from build123d import *

# Parameters (mm, degrees)
SKETCH2_R          = 4.445
CUT_EXTRUDE1_DEPTH = 18.034
CHAMFER1_SIZE      = 0.762
SKETCH5_W          = 11.240575932
SKETCH5_H          = 1.524
CUT_EXTRUDE2_DEPTH = 20.444017921
CIRPATTERN1_COUNT  = 4


with BuildPart() as part:
    # Sketch1 → Revolve1 (revolve)
    with BuildSketch(Plane.XY, mode=Mode.PRIVATE) as revolve1_sk:
        with BuildLine():
            Line((0, 0), (15.939575932, 0))
            Line((15.939575932, 0), (15.939575932, 6.251377289))
            ThreePointArc((15.939575932, 6.251377289), (15.12834599, 7.110581459), (14.224, 6.35))
            Line((14.224, 6.35), (1.524, 6.35))
            Line((1.524, 6.35), (1.524, 7.874))
            Line((1.524, 7.874), (0, 7.874))
            Line((0, 7.874), (0, 0))
        make_face()
    revolve(revolve1_sk.sketch.rotate(Axis((0, 0, 0), (1, 0, 0)), 90), axis=Axis((0, 0, 0), (1, 0, 0)))

    # Sketch2 → Cut-Extrude1 (cut)
    with BuildSketch(Plane.ZY):
        Circle(SKETCH2_R)
    extrude(amount=-CUT_EXTRUDE1_DEPTH, mode=Mode.SUBTRACT)

    # Chamfer1
    chamfer1_edges = [part.edges().sort_by_distance(p)[0] for p in [
        (15.939575932, 0, -4.445),
        (0, 0, -4.445),
    ]]
    chamfer(chamfer1_edges, length=CHAMFER1_SIZE)

    # Sketch5 → Cut-Extrude2 (cut, through all)
    with BuildSketch(Plane.XY):
        with Locations((10.319287966, 0)):
            Rectangle(SKETCH5_W, SKETCH5_H)
    cut_extrude2 = extrude(amount=-CUT_EXTRUDE2_DEPTH, mode=Mode.SUBTRACT)

    # CirPattern1: Cut-Extrude2 ×4 about axis
    cirpattern1_axis = Axis((0, 0, 0), (1, 0, 0))
    for i in range(1, CIRPATTERN1_COUNT):
        add(cut_extrude2.rotate(cirpattern1_axis, i * 360 / CIRPATTERN1_COUNT), mode=Mode.SUBTRACT)


solid = part.part
Can you work these out from the model? Positions are in its coordinate system, mm. A direction names the side the tool comes from. Give positions to 0.01 mm unless a question says otherwise; leave off trailing zeros. Order: outer loops, then holes, each group sorted by start corner. A loop starts at its lowest first (then second) coordinate and runs counter-clockwise, first axis right, second up. Notation, with made-up numbers: M -17,79 L 5,79 A23 ccw 5,101 Z; hole C 2,49 d10. An arc over 180 degrees is marked long. Use a Markdown table: item, result. Add a question column.
Item 1: For faces 1 (the flat face through (1.524, -6.5, -0.5)), 2 (the flat face through (15.94, 4, -4)), 3 (the flat face through (10, 5, -0.762)), 4 (the conical face through (15.4, 3.3, 3.3)), which set-ups out of +Z, -Z, +X, -X, +Y, -Y let a thin tool reach every point of the face, with its end or its side?
Item 2: Suppose I cut it at C-C (x = 6). List the corners of the cut face in (y, z) for me (3 decimals).
Item 3: Suppose I cut it at D-D (x = 2.5). List the corners of the cut face in (y, z) for me (3 decimals), then the cut area to 3 significant figures.
Item 4: We'd pull the mould along Y, two halves only. Please class faces 5 (the flat face through (15.94, 4, 4)), 6 (the cylindrical face through (7.785, -1.907, 6.057)), 7 (the flat face through (4.699, 0, -5)): +Y half, -Y half, draft (parallel to the pull), parting line (faces both ways), or undercut.
Item 5: Will these pins go through, and if not, where does the flat tip stop? pin 1 (6 mm diameter, centred on y = 1, z = -3.5, fed in from +X); pin 2 (1.3 mm diameter, centred on x = 10, y = -5.5, fed in from -Z); pin 3 (1.3 mm diameter, centred on x = 10, z = -5.5, fed in from +Y); pin 4 (2 mm diameter, centred on x = 11, z = 6.5, fed in from -Y).
Item 6: If I drill on L1, parallel to Y at x = 4.5, z = 0 (3 decimals); L2, parallel to Y at x = 3, z = 2.5; L3, parallel to Z at x = 7, y = -1.75, over which ranges is the centre line in solid material (lowest first)? Write a range as [from, to].
Item 7: Suppose I cut it at A-A (z = 0). List the corners of the cut face in (x, y) for me (3 decimals).
Answer sheet:
| question | item | result |
|---|---|---|
| 1 | face 1 | none |
| 1 | face 2 | +Z, -Z, +X, +Y, -Y |
| 1 | face 3 | +X, +Y, -Y |
| 1 | face 4 | +X |
| 2 | outline | M -6.304,-0.762 A6.35 ccw -0.762,-6.304 L -0.762,-4.379 A4.445 cw -4.379,-0.762 Z; M -6.304,0.762 L -4.379,0.762 A4.445 cw -0.762,4.379 L -0.762,6.304 A6.35 ccw Z; M 0.762,-6.304 A6.35 ccw 6.304,-0.762 L 4.379,-0.762 A4.445 cw 0.762,-4.379 Z; M 0.762,4.379 A4.445 cw 4.379,0.762 L 6.304,0.762 A6.35 ccw 0.762,6.304 Z |
| 3 | outline | C 0,0 d12.7; hole C 0,0 d8.89 |
| 3 | area | 64.6 mm² |
| 4 | face 5 | draft |
| 4 | face 6 | parting line |
| 4 | face 7 | undercut |
| 5 | pin 1 | stops at x = 15.94 |
| 5 | pin 2 | stops at z = -4.1 |
| 5 | pin 3 | stops at y = 4.1 |
| 5 | pin 4 | stops at y = -3.17 |
| 6 | L1 | y = [-6.35, -4.445], [4.445, 6.35] |
| 6 | L2 | y = [-5.84, -3.68], [3.68, 5.84] |
| 6 | L3 | z = [-6.1, -4.09], [4.09, 6.1] |
| 7 | outline | M 0,-7.874 L 1.524,-7.874 L 1.524,-6.35 L 4.699,-6.35 L 4.699,-4.445 L 0.762,-4.445 L 0,-5.207 Z; M 0,5.207 L 0.762,4.445 L 4.699,4.445 L 4.699,6.35 L 1.524,6.35 L 1.524,7.874 L 0,7.874 Z |
